Could you check a few things on this model? Use its own coordinates, in mm. Face numbers are marked on the shaded views. Round coordinates to 2 decimals unless told otherwise and drop trailing zeros. Write each loop counter-clockwise with the first axis right and the second up, starting at its lowest first coordinate (ties: lowest second). Pieces come first, ordered by that corner, then holes. Notation, with made-up numbers: (49.25, -37) -> (62.25, -37) arc R28 ccw to (62.25, -11) -> close; hole circle Ø9 at (43.25, -12.5). An arc over 180 degrees is marked (long way). Return JSON: item names as keys, results as strings.
from build123d import *

# Parameters (mm, degrees)
KES_EKSTR_ZYON1_DEPTH      = 35.641016151
KES_EKSTR_ZYON1_DEPTH_BACK = 35.641016151
M10_DI_LI_DELIK1_D         = 8.5
M10_DI_LI_DELIK1_DEPTH     = 10
M10_DI_LI_DELIK1_TIP       = 2.553657631


with BuildPart() as part:
    # Çizim1 → Döndür1 (revolve)
    with BuildSketch(Plane.XY):
        with BuildLine():
            Line((0, 20), (0, -20))
            ThreePointArc((0, -20), (20, 0), (0, 20))
        make_face()
    revolve(axis=Axis((0, 20, 0), (0, -1, 0)))

    # Çizim2 → Kes-Ekstrüzyon1 (cut, two sides: drawn at the far end of the back side and taken through both)
    with BuildSketch(Plane.XY.offset(-KES_EKSTR_ZYON1_DEPTH_BACK)):
        Polygon((-113.979792733, -18), (-8.717797887, -18), (8.717797887, -18), (113.979792733, -18), (113.979792733, -228.523989691), (-113.979792733, -228.523989691), align=None)
    extrude(amount=KES_EKSTR_ZYON1_DEPTH + KES_EKSTR_ZYON1_DEPTH_BACK, mode=Mode.SUBTRACT)

    # M10 Dişli Delik1
    with Locations(Plane(origin=(0, -18, 0), x_dir=(-1, 0, 0), z_dir=(0, -1, 0))):
        with Locations((0, 0)):
            Hole(M10_DI_LI_DELIK1_D / 2, depth=M10_DI_LI_DELIK1_DEPTH)
            with Locations((0, 0, -(M10_DI_LI_DELIK1_DEPTH + M10_DI_LI_DELIK1_TIP / 2))):  # 118° drill point
                Cone(0, M10_DI_LI_DELIK1_D / 2, M10_DI_LI_DELIK1_TIP, mode=Mode.SUBTRACT)


solid = part.part
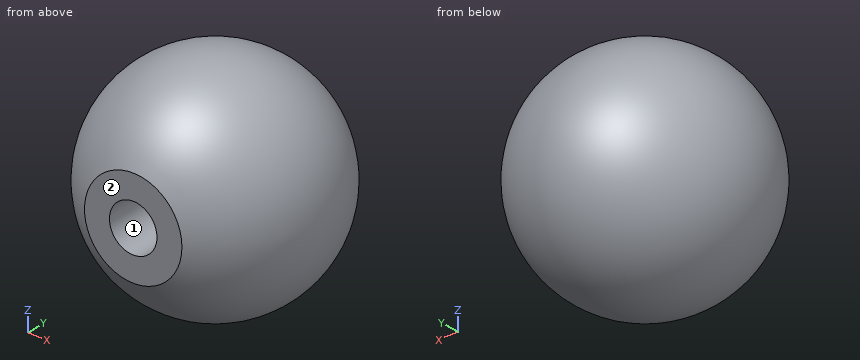
1) I want a section at A-A, the plane z = 17. Please give me the cut outline in (x, y), and give its area (3 significant figures).
Return value:
{"outline": "circle Ø21.07 at (0, 0)", "area": "349 mm²"}
2) Will these pins go through, and if not, where does the flat tip stop? pin 1 Ø2 at (x, y) = (-14, 9.5) entering from -Z; pin 2 Ø2 at (x, y) = (16, -0.5) entering from +Z; pin 3 Ø1.5 at (y, z) = (8, 16) entering from +X.
Return value:
{"pin 1": "z = -12.11", "pin 2": "z = 13.22", "pin 3": "x = 10.31"}
3) If I drill on probe 1 along Z at (x, y) = (0, -12.75); probe 2 along Z at (x, y) = (0, -15); probe 3 along X at (y, z) = (-9.5, 3), over which ranges is the centre line in solid material (lowest first)? Write a range as [from, to].
Return value:
{"probe 1": "[-15.41, -4.25], [4.25, 15.41]", "probe 2": "[-13.23, -4.25], [4.25, 13.23]", "probe 3": "[-17.34, -3.01], [3.01, 17.34]"}
4) I want a section at C-C, the plane y = -15. Please give me the cut outline in (x, z).
Return value:
{"outline": "circle Ø26.46 at (0, 0); hole circle Ø8.5 at (0, 0)"}
5) I want a section at B-B, the plane x = 14.5. Please give me the cut outline in (y, z), and give its area (3 significant figures).
Return value:
{"outline": "circle Ø27.55 at (0, 0)", "area": "596 mm²"}
6) I want a section at D-D, the plane x = -5.5. Please give me the cut outline in (y, z), and give its area (3 significant figures).
Return value:
{"outline": "(-18, -6.76) arc R19.23 ccw (long way) to (-18, 6.76) -> close", "area": "1,150 mm²"}
7) Thinking about a two-plate mould opening in Z: for the marked faces 1 and 2, which applies, pulls with the +Z half, pulls with the -Z half, needs draft (parallel to the pull), parting line crosses it, or undercut?
Return value:
{"face 1": "undercut", "face 2": "needs draft"}
